Study the drawing (mm; zero at the part's minimum x, y, z) and answer. A direction names the side the tool comes from. Give positions to 0.01 mm unless a question says otherwise; leave off trailing zeros. Write each loop counter-clockwise with the first axis right and the second up, starting at its lowest first coordinate (ties: lowest second). Pieces come first, ordered by that corner, then holes.
1) Given pin 1 Ø2 at (x, z) = (46.5, 4.5) entering from -Y; pin 2 Ø6 at (x, z) = (9, 1.5) entering from +Y; pin 3 Ø0.6 at (y, z) = (9.5, 4) entering from +X, each flat-ended and moving along its own axis, determine where each tip first touches the part or whether it passes through.
2) A tool of negligible diameter and unlimited length cuts with its end or side. For the marked faces 1, 2 and 3, from which of +Z, -Z, +X, -X, +Y, -Y can it reach the whole face along a straight path? Write none if from no direction.
3) Determine the mould class of the marked faces 4, 5, 6 and 7 for opening direction Y: pulls with the +Y half, pulls with the -Y half, needs draft (parallel to the pull), parting line crosses it, or undercut.
4) Straight lines are drawn through the part: probe 1 along X at (y, z) = (3, 5); probe 2 along X at (y, z) = (4.5, 6.75); probe 3 along X at (y, z) = (9.75, 3.75). For each, find the intervals that lie inside material, in ascending order.
5) Find section B-B (y = 5). Determine the outline of the cut face in (x, z).
6) Find section D-D (x = 42). Determine the outline of the cut face in (y, z).
7) Find section A-A (y = 11.5). Determine the outline of the cut face in (x, z), plus the area to 3 significant figures.
8) Find section C-C (x = 22). Determine the outline of the cut face in (y, z), plus the area to 3 significant figures.
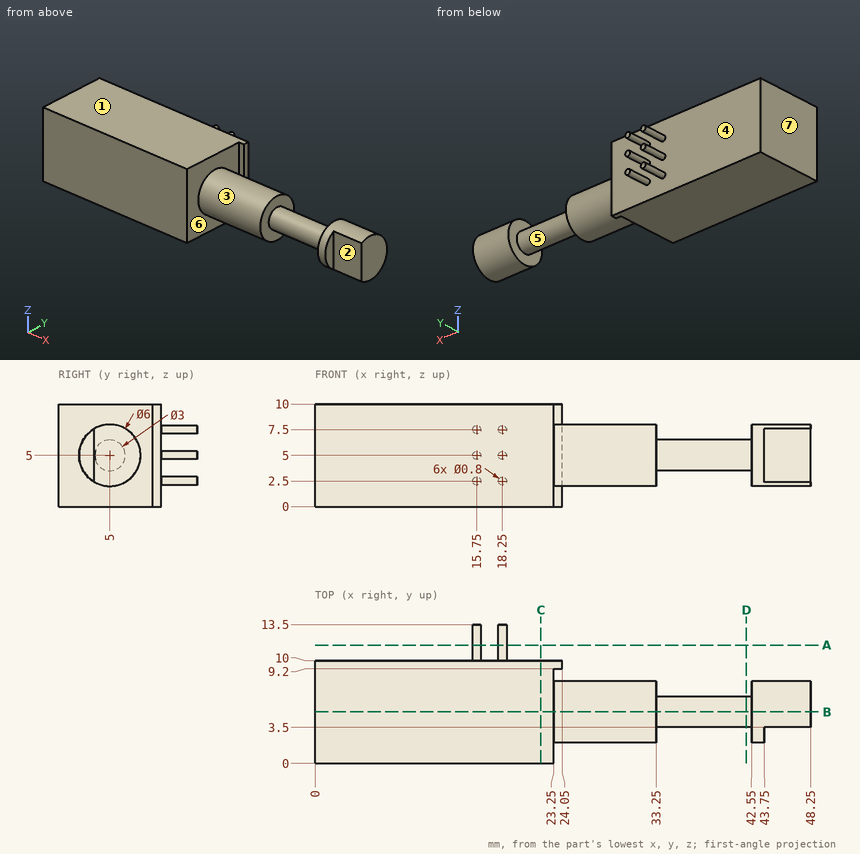
Results:
1. pin 1: stops at y = 3.5
1. pin 2: stops at y = 10
1. pin 3: stops at x = 24.05
2. face 1: +Z, +X, -X, +Y, -Y
2. face 2: +Z, -Z, +X, -Y
2. face 3: +X
3. face 4: pulls with the +Y half
3. face 5: parting line crosses it
3. face 6: undercut
3. face 7: needs draft
4. probe 1: x = 0 to 33.25, 42.55 to 43.75
4. probe 2: x = 0 to 33.25, 42.55 to 48.25
4. probe 3: x = 0 to 24.05
5. outline: (0, 0) - (23.25, 0) - (23.25, 2) - (33.25, 2) - (33.25, 3.5) - (42.55, 3.5) - (42.55, 2) - (48.25, 2) - (48.25, 8) - (42.55, 8) - (42.55, 6.5) - (33.25, 6.5) - (33.25, 8) - (23.25, 8) - (23.25, 10) - (0, 10) - close
6. outline: circle Ø3 at (5, 5)
7. outline: circle Ø0.8 at (15.75, 2.5); circle Ø0.8 at (15.75, 5); circle Ø0.8 at (15.75, 7.5); circle Ø0.8 at (18.25, 2.5); circle Ø0.8 at (18.25, 5); circle Ø0.8 at (18.25, 7.5)
7. area: 3.02 mm2
8. outline: (0, 0) - (10, 0) - (10, 10) - (0, 10) - close
8. area: 100 mm2
